Input: dimensioned drawing with shaded views. Units: mm. Origin: part minimum x, y, z. A direction names the side the tool comes from. Give positions to 0.01 mm unless a question says otherwise; leave off trailing zeros. Write each loop counter-clockwise with the first axis right and the second up, starting at its lowest first coordinate (ties: lowest second). Pieces come first, ordered by that corner, then holes.
Q1. Section A-A (x = 2.8). Return the cut outline in (y, z).
Q2. Section C-C (y = 1.5). Return the cut outline in (x, z).
Q3. Section B-B (z = 2.8). Return the cut outline in (x, y).
Q4. Line query: line 1 (Y direction, x = 3.85, z = 2.9); line 2 (Y direction, x = 4, z = 1.15); line 3 (Z direction, x = 1.7, y = 1) (1 decimal). Output: solid intervals per line, ascending.
Q5. Reachability of the marked faces 1, 2 and 3 from +Z, -Z, +X, -X, +Y, -Y: full face, straight path, thin tool, end or side. Return the list, or none.
Q6. Section D-D (y = 7.25). Return the cut outline in (x, z), plus the area to 3 significant figures.
Q7. Pin query (flat end, axial travel): pin 1 Ø0.6 at (x, y) = (2, 0.5) entering from +Z (1 decimal); pin 2 Ø1.5 at (x, y) = (4.5, 8.5) entering from +Z; pin 3 Ø0.6 at (x, z) = (2, 2.5) entering from -Y. Return the tip coordinate at first contact, or that it passes through.
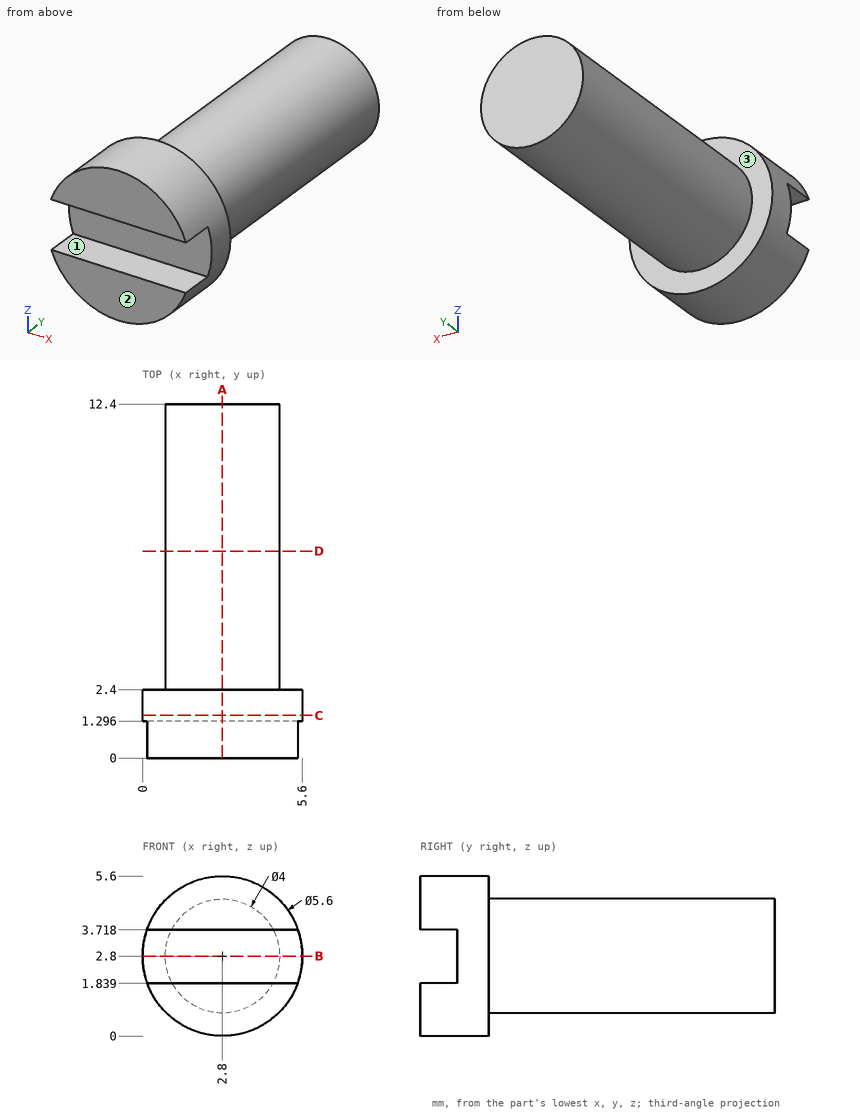
Computed:
1. outline: (0, 0) - (2.4, 0) - (2.4, 0.8) - (12.4, 0.8) - (12.4, 4.8) - (2.4, 4.8) - (2.4, 5.6) - (0, 5.6) - (0, 3.72) - (1.3, 3.72) - (1.3, 1.84) - (0, 1.84) - close
2. outline: circle Ø5.6 at (2.8, 2.8)
3. outline: (0, 1.3) - (5.6, 1.3) - (5.6, 2.4) - (4.8, 2.4) - (4.8, 12.4) - (0.8, 12.4) - (0.8, 2.4) - (0, 2.4) - close
4. line 1: y = 1.3 to 12.4
4. line 2: y = 0 to 2.4
4. line 3: z = 0.2 to 1.8, 3.7 to 5.4
5. face 1: +X, -X, -Y
5. face 2: +Z, -Z, +X, -X, -Y
5. face 3: +Y
6. outline: circle Ø4 at (2.8, 2.8)
6. area: 12.6 mm2
7. pin 1: stops at z = 5.6
7. pin 2: stops at z = 4.56
7. pin 3: stops at y = 1.3
